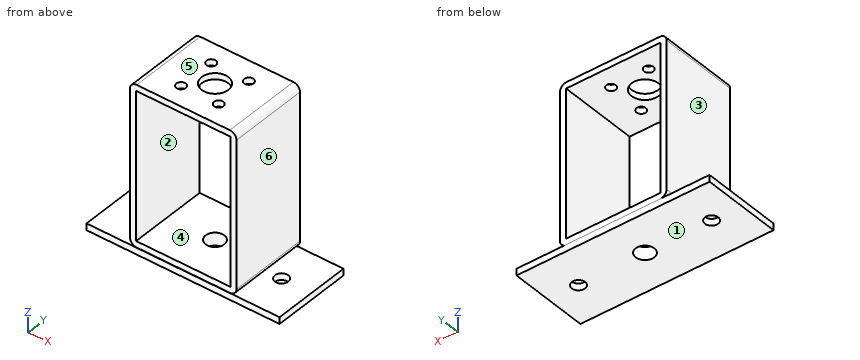
from build123d import *

# Parameters (mm, degrees)
F0_W     = 89.916
F0_H     = 140.716
F1_DEPTH = 37.846
F2_R     = 4.4704
F2_R_2   = 12.7
F3_DEPTH = 25.4
F4_W     = 184.15
F4_H     = 76.2
F4_W_2   = 88.9
F4_H_2   = 75.692
F5_DEPTH = 6.35
F6_R     = 6.35
F6_R_2   = 8.89
F7_DEPTH = 25.4


with BuildPart() as f1:
    # F0 (on Front) → F1 (new body, symmetric)
    with BuildSketch(Plane.XZ):
        with BuildLine():
            Line((44.45, 76.2), (-44.45, 76.2))
            ThreePointArc((-44.45, 76.2), (-48.9401280605, 74.3401280605), (-50.8, 69.85))
            Line((-50.8, 69.85), (-50.8, -69.85))
            ThreePointArc((-50.8, -69.85), (-48.9401280605, -74.3401280605), (-44.45, -76.2))
            Line((-44.45, -76.2), (44.45, -76.2))
            ThreePointArc((44.45, -76.2), (48.9401280605, -74.3401280605), (50.8, -69.85))
            Line((50.8, -69.85), (50.8, 69.85))
            ThreePointArc((50.8, 69.85), (48.9401280605, 74.3401280605), (44.45, 76.2))
        make_face()
        Rectangle(F0_W, F0_H, mode=Mode.SUBTRACT)
    extrude(amount=F1_DEPTH, both=True)

    # F2 (on face) → F3 (cut)
    with BuildSketch(Plane.XY.offset(76.2)):
        with Locations((-17.96034, 17.96034)):
            Circle(F2_R)
        with Locations((17.96034, 17.96034)):
            Circle(F2_R)
        with Locations((17.96034, -17.96034)):
            Circle(F2_R)
        with Locations((-17.96034, -17.96034)):
            Circle(F2_R)
        Circle(F2_R_2)
    extrude(amount=-F3_DEPTH, mode=Mode.SUBTRACT)

    # F4 (on face) → F5 (join)
    with BuildSketch(Plane(origin=(0, 0, -76.2), x_dir=(1, 0, 0), z_dir=(0, 0, -1))):
        Rectangle(F4_W, F4_H)
        Rectangle(F4_W_2, F4_H_2, mode=Mode.SUBTRACT)
        Rectangle(F4_W_2, F4_H_2)
    extrude(amount=F5_DEPTH)

    # F6 (on face) → F7 (cut)
    with BuildSketch(Plane(origin=(0, 0, -82.55), x_dir=(1, 0, 0), z_dir=(0, 0, -1))):
        with Locations((63.5, 0)):
            Circle(F6_R)
        Circle(F6_R_2)
        with Locations((-63.5, 0)):
            Circle(F6_R)
    extrude(amount=-F7_DEPTH, mode=Mode.SUBTRACT)


solid = f1.part
Design review of the part built by this model. Coordinates are the model's own, in mm. Face numbers are marked on the shaded views. A direction names the side the tool comes from. Round coordinates to 2 decimals unless told otherwise and drop trailing zeros. Loops run counter-clockwise (first coordinate to the right, second up) from the corner with the lowest first, then second, coordinate; pieces in that order, holes last. Notation, with made-up numbers: (-16.75, 89) - (-8.75, 89) arc R32 cw to (-8.75, 120) - close; hole circle Ø7 at (-37, 36). An arc over 180 degrees is marked (long way). One line per question, with ' | ' between items.
1. For the marked faces 1, 2 and 3, list the 3-axis set-ups (+Z, -Z, +X, -X, +Y, -Y) from which the entire face can be reached by the end or side of a thin tool; tool diameter is ignored.
Results are:
face 1: -Z, +X, -X, +Y, -Y | face 2: +Y, -Y | face 3: +Z, -X, +Y, -Y
2. Clearance check with flat-ended pins moving along their axes: P1, Ø20.5, axis at x = -63.5, y = 0, coming from the -Z side; P2, Ø6, axis at x = 67.5, y = 20, coming from the +Z side; P3, Ø3, axis at y = 20, z = 53, coming from the -X side; P4, Ø5.5, axis at x = -17.96, y = 17.96, coming from the +Z side. State where each tip first meets the part, or that it passes through.
Results are:
P1: stops at z = -82.55 | P2: stops at z = -76.2 | P3: stops at x = -50.8 | P4: stops at z = -70.36
3. We need section B-B, the plane y = 0. State how many separate pieces and enclosed holes the cut face has, and give its area (3 significant figures).
Results are:
separate pieces: 4 | enclosed holes: 0 | area: 3,440 mm²
4. For L1, parallel to X at y = 0, z = -77.5 (3 decimals); L2, parallel to X at y = 22, z = -61; L3, parallel to Z at x = -15, y = 26, list the stretches that pass through material, from the lowest coordinate up. Write a range as [from, to].
Results are:
L1: x = [-92.075, -69.85], [-57.15, -8.89], [8.89, 57.15], [69.85, 92.075] | L2: x = [-50.8, -44.96], [44.96, 50.8] | L3: z = [-82.55, -70.36], [70.36, 76.2]
5. We need section D-D, the plane y = -27.5. State the section outline as (x, z) points (3 decimals).
Results are:
outline: (-92.075, -82.55) - (92.075, -82.55) - (92.075, -76.2) - (44.45, -76.2) arc R6.35 ccw to (50.8, -69.85) - (50.8, 69.85) arc R6.35 ccw to (44.45, 76.2) - (-44.45, 76.2) arc R6.35 ccw to (-50.8, 69.85) - (-50.8, -69.85) arc R6.35 ccw to (-44.45, -76.2) - (-92.075, -76.2) - close; hole (-44.958, -70.358) - (44.958, -70.358) - (44.958, 70.358) - (-44.958, 70.358) - close
6. We need section A-A, the plane z = 50. State the section outline as (x, y) points, and give its area (3 significant figures).
Results are:
outline: (-50.8, -37.85) - (-44.96, -37.85) - (-44.96, 37.85) - (-50.8, 37.85) - close; (44.96, -37.85) - (50.8, -37.85) - (50.8, 37.85) - (44.96, 37.85) - close | area: 884 mm²
7. Draft analysis for pull direction X (two halves, no side actions). For the marked faces 4, 5 and 6, state which applies: released by +X, released by -X, zero draft, split by the parting line, or undercut.
Results are:
face 4: undercut | face 5: zero draft | face 6: released by +X
8. We need section C-C, the plane x = 63.5. State the section outline as (y, z) points, and give its area (3 significant figures).
Results are:
outline: (-38.1, -82.55) - (-6.35, -82.55) - (-6.35, -76.2) - (-38.1, -76.2) - close; (6.35, -82.55) - (38.1, -82.55) - (38.1, -76.2) - (6.35, -76.2) - close | area: 403 mm²
